Check sheet for the drawn part. Datum: minimum x, y, z corner. Units: mm. Round coordinates to 2 decimals unless told otherwise and drop trailing zeros. Order: outer loops, then holes, each group sorted by start corner. A loop starts at its lowest first (then second) coordinate and runs counter-clockwise, first axis right, second up. Notation, with made-up numbers: M 38.5,44.5 L 58.5,44.5 A24 cw 58.5,81.5 Z; hole C 2.25,78 d6. An arc over 180 degrees is marked long. Answer as a JSON object with one key per item and string values. Group by question number.
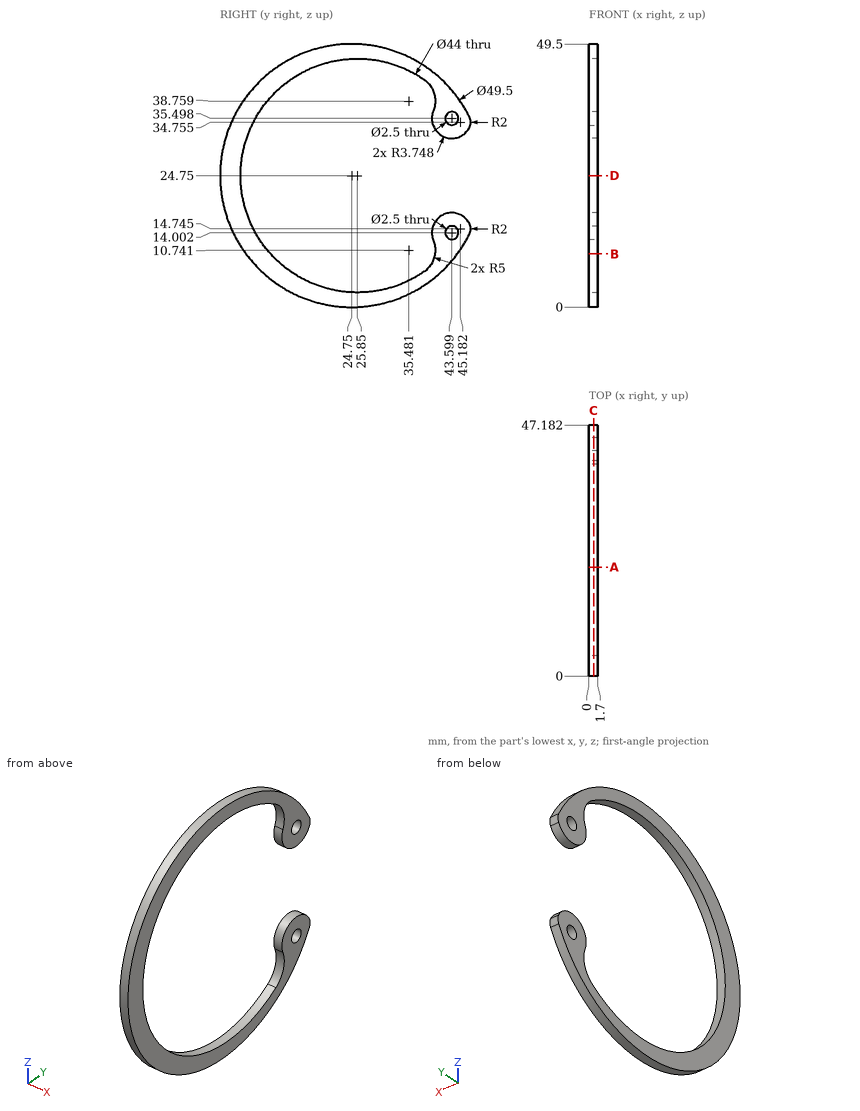
1) Sectioned sample at C-C (x = 0.9). Count the separate pieces of the cut face and the enclosed holes in it.
2) Sectioned sample at A-A (y = 20.5). Record the boundary of the cut face in (x, z).
3) Sectioned sample at B-B (z = 10). Record the boundary of the cut face in (x, y) (1 decimal).
4) Sectioned sample at D-D (z = 24.75). Record the boundary of the cut face in (x, y).
5) Go/stop test with a flat-tipped pin: P1, Ø4, axis at y = 43.6, z = 14, coming from the -X side. Record where the tip stops, or that it passes through.
6) Thickness scan on line 1 along Y through (x, z) = (0.95, 39.5) (1 decimal); line 2 along Z through (x, y) = (1.3, 24.5); line 3 along Z through (x, y) = (0.1, 34) (1 decimal). Record the ranges inside material, lowest first. Write a range as [from, to].
Final values:
{
 "1": {"separate pieces": "1", "enclosed holes": "2"},
 "2": {"outline": "M 0,0.37 L 1.7,0.37 L 1.7,3.41 L 0,3.41 Z; M 0,46.09 L 1.7,46.09 L 1.7,49.13 L 0,49.13 Z"},
 "3": {"outline": "M 0,4.9 L 1.7,4.9 L 1.7,9.5 L 0,9.5 Z; M 0,40.4 L 1.7,40.4 L 1.7,44.6 L 0,44.6 Z"},
 "4": {"outline": "M 0,0 L 1.7,0 L 1.7,3.85 L 0,3.85 Z"},
 "5": {"P1": "stops at x = 0"},
 "6": {"line 1": "y = [4.9, 9.5], [40.4, 44.6]", "line 2": "z = [0, 2.79], [46.71, 49.5]", "line 3": "z = [1.8, 4.3], [45.2, 47.7]"}
}
